Autodesk Inventor part; units mm, degrees
ref_plane "YZ Plane" through (0, 0, 0) normal (1, 0, 0) x (0, 1, 0)
ref_plane "XZ Plane" through (0, 0, 0) normal (0, 1, 0) x (-1, 0, 0)
ref_plane "XY Plane" through (0, 0, 0) normal (0, 0, 1) x (1, 0, 0)
sketch "Sketch1" plane through (0, 0, 0) normal (0, 1, 0) x (-1, 0, 0)
  line L0 (0, 0) -> (76.2, 0)
  line L1 (76.2, 0) -> (76.2, -38.1)
  line L2 (76.2, -38.1) -> (0, -38.1)
  line L3 (0, -38.1) -> (0, 0)
  dimension "d0" = 76.2
  dimension "d1" = 38.1
extrude "Plate1" add sketch "Sketch1" along normal blind 6.35
sketch "Sketch2" plane through (0, 6.35, 0) normal (0, 1, 0) x (1, 0, 0)
  line L0 (-76.2, 38.1) -> (0, 38.1)
  line L1 (-76.2, 0) -> (-76.2, 38.1)
  point P0 (0, 0)
  point P1 (-38.1, 19.05)
  dimension "d3" = 19.05
  dimension "d4" = 38.1
hole "Hole1" at (-38.1, 6.35, -19.05) direction (0, -1, 0) diameter 28.575 end through all
sketch "Sketch4" plane through (0, 6.35, 0) normal (0, 1, 0) x (1, 0, 0)
  line L0 (-66.675, 19.05) -> (-9.525, 19.05) construction
  circle A0 centre (-38.1, 19.05) radius 14.2875 construction
  point P0 (0, 0)
  dimension "d28" = 28.575
  dimension "d29" = 28.575
hole "Hole3" at (-66.675, 6.35, -19.05) at (-9.525, 6.35, -19.05) direction (0, -1, 0) diameter 6.5278 end through all
equation "\"d10\" = Thickness"
equation "\"d28\" = CenterPointToTensionerRound"
equation "\"d29\" = d28"
equation "\"d31\" = ShapeWidth"
equation "\"d35\" = Thickness"
equation "\"d2\" = Thickness"
equation "\"BendRadius\" = 1.5 * Thickness"
equation "\"BendReliefWidth\" = Thickness"
equation "\"BendReliefDepth\" = 0.5 * Thickness"
equation "\"CornerReliefSize\" = 4 * Thickness"
equation "\"MinimumRemnant\" = 2 * Thickness"
equation "\"TransitionRadius\" = BendRadius"
equation "\"JacobiRadiusSize\" = BendRadius"
equation "\"GapSize\" = Thickness"
equation "\"DrivebaseLength\" = 762"
equation "\"DrivebaseWidth\" = 660.4"
equation "\"CenterlineDrivebaseLength\" = 736.6"
equation "\"CenterlineDrivebaseWidth\" = 635"
equation "\"ShapeHeight\" = 76.2"
equation "\"ShapeWidth\" = 25.4"
equation "\"ShapeThickness\" = 3.175"
equation "\"WheelDiameter\" = 152.4"
equation "\"WheelRadius\" = 76.2"
equation "\"WheelClearancetoFrame\" = 25.4"
equation "\"WheelDistanceFromEdge\" = 101.6"
equation "\"SlotLength\" = 88.9"
equation "\"SlotWidth\" = 15.9512"
equation "\"CenterAxleDrop\" = 3.175"
equation "\"SlidingTensionerRoundDiameter\" = 15.875"
equation "\"SlidingTensionerRoundClearance\" = 0.0762"
equation "\"CenterAxleXPosition\" = 381"
equation "\"CenterAxleYPosition\" = 25.4"
equation "\"Crossmember1Position\" = 203.2"
equation "\"Crossmember2Position\" = 203.2"
equation "\"TensionAssemblyJointTravelLengthStart\" = -15.875"
equation "\"TensionAssemblyJointTravelLengthEnd\" = 15.875"
equation "\"CenterPointToTensionerRound\" = 28.575"
properties part number "200288" material "Aluminum 5052 H32"
Can you work these out from the model? Positions are in its coordinate system, mm. Give positions to 0.01 mm unless a question says otherwise; leave off trailing zeros. Loops run counter-clockwise (first coordinate to the right, second up) from the corner with the lowest first, then second, coordinate; pieces in that order, holes last. Notation, with made-up numbers: (86, 19) -> (95, 19) arc R18 cw to (95, 45) -> close; hole circle Ø1 at (-23.5, 16.25). An arc over 180 degrees is marked (long way). Return JSON: item names as keys, results as strings.
Q1. I want a section at A-A, the plane z = -19.05. List the corners of the cut face in (x, y) for me.
Checks:
{"outline": "(-76.2, 0) -> (-69.94, 0) -> (-69.94, 6.35) -> (-76.2, 6.35) -> close; (-63.41, 0) -> (-52.39, 0) -> (-52.39, 6.35) -> (-63.41, 6.35) -> close; (-23.81, 0) -> (-12.79, 0) -> (-12.79, 6.35) -> (-23.81, 6.35) -> close; (-6.26, 0) -> (0, 0) -> (0, 6.35) -> (-6.26, 6.35) -> close"}
Q2. For pin 1 Ø5 at (x, z) = (-66.675, -19.05) entering from +Y, with a flat end and sliding along its axis, tell me the tip position at first contact or that it passes through.
Checks:
{"pin 1": "passes through"}
Q3. I want a section at B-B, the plane x = -38.1. List the corners of the cut face in (y, z) for me, then the cut area to 3 significant figures.
Checks:
{"outline": "(0, -38.1) -> (6.35, -38.1) -> (6.35, -33.34) -> (0, -33.34) -> close; (0, -4.76) -> (6.35, -4.76) -> (6.35, 0) -> (0, 0) -> close", "area": "60.5 mm2"}
Q4. I want a section at C-C, the plane z = -28. List the corners of the cut face in (x, y) for me, then the cut area to 3 significant figures.
Checks:
{"outline": "(-76.2, 0) -> (-49.24, 0) -> (-49.24, 6.35) -> (-76.2, 6.35) -> close; (-26.96, 0) -> (0, 0) -> (0, 6.35) -> (-26.96, 6.35) -> close", "area": "342 mm2"}
Q5. We'd pull the mould along X, two halves only. Please class faces 1 (the face through (-76.2, 3, -19)), 2 (the face through (-68.881, 3.131, -21.456)), 3 (the face through (-46, 0, -31.5)): released by +X, released by -X, zero draft, split by the parting line, or undercut.
Checks:
{"face 1": "released by -X", "face 2": "undercut", "face 3": "zero draft"}
Q6. I need wall thicknesses on probe 1 along X at (y, z) = (3, -19.05); probe 2 along Z at (x, y) = (-38.1, 2); probe 3 along Z at (x, y) = (-12, 3). Which ranges of each line are inside material? Lowest first, please.
Checks:
{"probe 1": "x = -76.2 to -69.94, -63.41 to -52.39, -23.81 to -12.79, -6.26 to 0", "probe 2": "z = -38.1 to -33.34, -4.76 to 0", "probe 3": "z = -38.1 to -21.18, -16.92 to 0"}
Q7. I want a section at D-D, the plane y = 3. Count the separate pieces of the cut face and the enclosed holes in it, then the cut area to 3 significant figures.
Checks:
{"separate pieces": "1", "enclosed holes": "3", "area": "2,190 mm2"}
